Source: CAD feature listing. Evaluate the final solid. Frame: model axes, mm. Face numbers are marked on the shaded views. A direction names the side the tool comes from. Give positions to 0.01 mm unless a question says otherwise; leave off trailing zeros. Loops run counter-clockwise (first coordinate to the right, second up) from the corner with the lowest first, then second, coordinate; pieces in that order, holes last. Notation, with made-up numbers: (59, 77) -> (75, 77) arc R14 ccw to (75, 85) -> close; hole circle Ø9 at (18.25, 9.25). An arc over 180 degrees is marked (long way). Return JSON: item names as keys, results as strings. Group by question number.
(1) Cut plane D-D on z = 7. Return loops of the section in (x, y) (1 decimal), then the cut area to 3 significant figures.
(2) Pin query (flat end, axial travel): pin 1 (4 mm diameter, centred on x = 1.5, y = 68, fed in from -Z); pin 2 (1 mm diameter, centred on x = 64, z = 56, fed in from -Y); pin 3 (11 mm diameter, centred on x = 65.5, y = -5.5, fed in from -Z); pin 4 (4 mm diameter, centred on x = 77.5, y = -23, fed in from +Z). Return the tip coordinate at first contact, or that it passes through.
(3) Cut plane C-C on x = 42.5. Return loops of the section in (y, z), then the cut area to 3 significant figures.
(4) Draft query along Y for the marked faces 4, 5 and 6. Return one class per face: released by +Y, released by -Y, zero draft, split by the parting line, or undercut.
(5) Ray query, line 1 (X direction, y = 0, z = 19.5); line 2 (X direction, y = 0, z = 63.5). Return the intervals inside material, ascending. Write a range as from..to.
(6) Access query for the marked faces 1, 2 and 3. Directions: +Z, -Z, +X, -X, +Y, -Y. A direction counts if a zero-diameter tool reaches every point of the face in a straight line with its end or side. Return the directions, or none.
```python
from build123d import *

# Parameters (mm, degrees)
F2_R     = 7
F3_DEPTH = 61.8


with BuildPart() as f1:
    # F0 (on Front) → F1 (revolve)
    with BuildSketch(Plane.XZ):
        Polygon((-84.75, 0), (-19.9375, 0), (-19.9375, 83.8), (-24.225, 83.8), (-24.225, 63.8), (-84.75, 63.8), (-84.75, 11.5), (-139, 11.5), (-139, 2), (-84.75, 2), align=None)
    revolve(axis=Axis((0, 0, 41.9), (0, 0, 1)))

    # F2 (on Top) → F3 (cut)
    with BuildSketch(Plane.XY):
        with Locations((64.957023, -2.363298)):
            Circle(F2_R)
        with Locations((2.363298, 64.957023)):
            Circle(F2_R)
        with Locations((-64.957023, 2.363298)):
            Circle(F2_R)
        with Locations((-2.363298, -64.957023)):
            Circle(F2_R)
    extrude(amount=F3_DEPTH, mode=Mode.SUBTRACT)


solid = f1.part
```
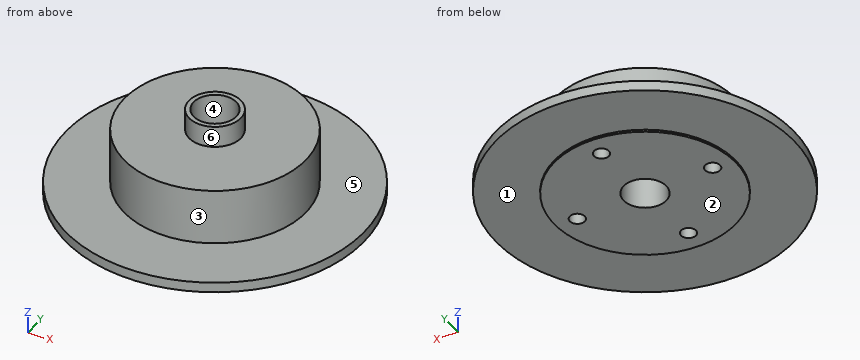
Answers:
{
 "1": {"outline": "circle Ø278 at (0, 0); hole circle Ø14 at (-65, 2.4); hole circle Ø39.9 at (0, 0); hole circle Ø14 at (-2.4, -65); hole circle Ø14 at (2.4, 65); hole circle Ø14 at (65, -2.4)", "area": "58,800 mm²"},
 "2": {"pin 1": "z = 61.8", "pin 2": "y = -56.13", "pin 3": "z = 0", "pin 4": "z = 63.8"},
 "3": {"outline": "(-132.34, 2) -> (-73.32, 2) -> (-73.32, 0) -> (73.32, 0) -> (73.32, 2) -> (132.34, 2) -> (132.34, 11.5) -> (73.32, 11.5) -> (73.32, 63.8) -> (-73.32, 63.8) -> (-73.32, 11.5) -> (-132.34, 11.5) -> close", "area": "10,500 mm²"},
 "4": {"face 4": "undercut", "face 5": "zero draft", "face 6": "split by the parting line"},
 "5": {"line 1": "-84.75..-71.55, -58.37..-19.94, 19.94..58.37, 71.55..84.75", "line 2": "-84.75..-19.94, 19.94..84.75"},
 "6": {"face 1": "-Z", "face 2": "-Z, +X, -X, +Y, -Y", "face 3": "+Z"}
}
